Check sheet for the modelled part. Datum: model origin and axes. Units: mm. A direction names the side the tool comes from. Give positions to 0.01 mm unless a question says otherwise; leave off trailing zeros. Loops run counter-clockwise (first coordinate to the right, second up) from the corner with the lowest first, then second, coordinate; pieces in that order, holes last. Notation, with made-up numbers: (-23, 43.5) -> (17, 43.5) arc R16 cw to (17, 70.5) -> close; hole circle Ø6 at (84, 15). An arc over 180 degrees is marked (long way). Write each question's results on one line, items separated by ' | '. Start each with the question number.
1. Mould release check, pull along X, two halves, no side actions. Record for faces 5 (the face through (49.226, 17, 28)), 6 (the face through (-55.774, 17, 27)), 7 (the face through (57, 27, 21)): +X half, -X half, draft (parallel to the pull), parting line (faces both ways), or undercut.
2. Gauge pin test, flat ends, axial feed: pin 1 Ø4 at (x, z) = (39.5, 28.5) entering from -Y; pin 2 Ø8 at (x, y) = (-5.5, 0) entering from -Z; pin 3 Ø5.5 at (x, z) = (-7, 28.5) entering from +Y. Record the tip position at first contact, or that the pin passes through.
3. Cross-section at C-C on y = -7. Record the boundary of the cut face in (x, z), and give its area (3 significant figures).
4. Cross-section at A-A on y = 22.5. Record the boundary of the cut face in (x, z), and give its area (3 significant figures).
5. Cross-section at D-D on x = 25.5. Record the boundary of the cut face in (y, z).
6. Cross-section at B-B on z = 15. Record the boundary of the cut face in (x, y), and give its area (3 significant figures).
7. Tool access check on faces 1 (the face through (-40.774, 18, 27)), 2 (the face through (45, 0, 29)), 3 (the face through (4.08, -6.06, 32.48)), 4 (the face through (57, 25, 19)). Record the directions out of +Z, -Z, +X, -X, +Y, -Y that give a thin tool (end or side, any length) a straight path to the whole face; none if there is none.
8. Material ranges on L1, parallel to X at y = 10, z = 30; L2, parallel to Z at x = 22.5, y = -8; L3, parallel to Y at x = 7.5, z = 41, recorded low to high. Write a range as from..to.
from build123d import *

# Parameters (mm, degrees)
SKETCH_1_W          = 120
SKETCH_1_H          = 5
EXTRUDE_1_DEPTH     = 3
SKETCH_2_W          = 15
SKETCH_2_H          = 5
EXTRUDE_2_DEPTH     = 24
SKETCH_3_W          = 50
SKETCH_3_H          = 30
EXTRUDE_3_DEPTH     = 10
FILLET_6_R          = 1
FILLET_7_R          = 5
FILLET_9_R          = 2
FILLET_10_R         = 2
CUT_EXTRUDE_1_DEPTH = 8
SKETCH_5_W          = 15
SKETCH_5_H          = 2
EXTRUDE_4_DEPTH     = 16


with BuildPart() as part:
    # 草图1 → 凸台-拉伸1 (new body)
    with BuildSketch(Plane(origin=(0, 0, 0), x_dir=(1, 0, 0), z_dir=(0, 1, 0))):
        with Locations((4.226022422, -28.977588204)):
            Rectangle(SKETCH_1_W, SKETCH_1_H)
    extrude(amount=EXTRUDE_1_DEPTH)

    # 草图2 → 凸台-拉伸2 (add)
    with BuildSketch(Plane(origin=(0, 3, 0), x_dir=(1, 0, 0), z_dir=(0, 1, 0))):
        with Locations((-48.273977578, -28.977588204)):
            Rectangle(SKETCH_2_W, SKETCH_2_H)
        with Locations((56.726022422, -28.977588204)):
            Rectangle(SKETCH_2_W, SKETCH_2_H)
    extrude(amount=EXTRUDE_2_DEPTH)

    # 草图3 → 凸台-拉伸3 (add)
    with BuildSketch(Plane.XZ):
        with Locations((4.226022422, 41.477588204)):
            Rectangle(SKETCH_3_W, SKETCH_3_H)
    extrude(amount=EXTRUDE_3_DEPTH)

    # 圆角6
    fillet_6_edges = [part.edges().sort_by_distance(p)[0] for p in [
        (4.226022422, 0, 31.477588204),
    ]]
    fillet(fillet_6_edges, radius=FILLET_6_R)

    # 圆角7
    fillet_7_edges = [part.edges().sort_by_distance(p)[0] for p in [
        (4.226022422, 0, 56.477588204),
    ]]
    fillet(fillet_7_edges, radius=FILLET_7_R)

    # 圆角9
    fillet_9_edges = [part.edges().sort_by_distance(p)[0] for p in [
        (64.226022422, 0, 28.977588204),
    ]]
    fillet(fillet_9_edges, radius=FILLET_9_R)

    # 圆角10
    fillet_10_edges = [part.edges().sort_by_distance(p)[0] for p in [
        (-55.773977578, 0, 28.977588204),
    ]]
    fillet(fillet_10_edges, radius=FILLET_10_R)

    # 草图4 → 切除-拉伸1 (cut)
    with BuildSketch(Plane.XZ.offset(10)):
        with BuildLine():
            ThreePointArc((-4.093422023, 38.044390841), (4.226022422, 32.477588204), (12.545466866, 38.044390841))
            ThreePointArc((12.545466866, 38.044390841), (16.726022422, 41.477588204), (12.545466866, 44.910785567))
            ThreePointArc((12.545466866, 44.910785567), (4.226022422, 50.477588204), (-4.093422023, 44.910785567))
            ThreePointArc((-4.093422023, 44.910785567), (-8.273977578, 41.477588204), (-4.093422023, 38.044390841))
        make_face()
    extrude(amount=-CUT_EXTRUDE_1_DEPTH, mode=Mode.SUBTRACT)

    # 草图5 → 凸台-拉伸4 (add)
    with BuildSketch(Plane(origin=(0, 0, 26.477588204), x_dir=(-1, 0, 0), z_dir=(0, 0, -1))):
        with Locations((-56.726022422, 26)):
            Rectangle(SKETCH_5_W, SKETCH_5_H)
        with Locations((48.273977578, 26)):
            Rectangle(SKETCH_5_W, SKETCH_5_H)
    extrude(amount=EXTRUDE_4_DEPTH)


solid = part.part
Geometry says:
1) face 5: undercut | face 6: -X half | face 7: draft
2) pin 1: y = 0 | pin 2: z = 26.48 | pin 3: y = 3
3) outline: (-20.77, 26.48) -> (29.23, 26.48) -> (29.23, 56.48) -> (-20.77, 56.48) -> close; hole (-4.09, 38.04) arc R9 ccw to (12.55, 38.04) arc R3.5 ccw (long way) to (12.55, 44.91) arc R9 ccw to (-4.09, 44.91) arc R3.5 ccw (long way) to start | area: 1,200 mm^2
4) outline: (-55.77, 26.48) -> (-40.77, 26.48) -> (-40.77, 31.48) -> (-55.77, 31.48) -> close; (49.23, 26.48) -> (64.23, 26.48) -> (64.23, 31.48) -> (49.23, 31.48) -> close | area: 150 mm^2
5) outline: (-10, 26.48) -> (3, 26.48) -> (3, 31.48) -> (1, 31.48) arc R1 cw to (0, 32.48) -> (0, 51.48) arc R5 ccw to (-5, 56.48) -> (-10, 56.48) -> close
6) outline: (-55.77, 25) -> (-40.77, 25) -> (-40.77, 27) -> (-55.77, 27) -> close; (49.23, 25) -> (64.23, 25) -> (64.23, 27) -> (49.23, 27) -> close | area: 60.0 mm^2
7) face 1: +Z, -Z, +Y | face 2: +Z, -Z, +X, -Y | face 3: -Y | face 4: -Z, +X, -X, -Y
8) L1: -55.77..-40.77, 49.23..64.23 | L2: 26.48..56.48 | L3: -2..0
